Could you check a few things on this model? Use its own coordinates, in mm. A direction names the side the tool comes from. Give positions to 0.01 mm unless a question says otherwise; leave off trailing zeros. Loops run counter-clockwise (first coordinate to the right, second up) from the corner with the lowest first, then second, coordinate; pieces in that order, holes last. Notation, with made-up numbers: (62, 28.25) -> (99, 28.25) arc R19 ccw to (99, 55.25) -> close; hole circle Ø5 at (89.5, 16.25). An arc over 180 degrees is marked (long way). Put each result on its own line as item: value.
```python
from build123d import *

# Parameters (mm, degrees)
SKETCH_1_W          = 130
SKETCH_1_H          = 62
EXTRUDE_1_DEPTH     = 3
SKETCH_2_R          = 2.6
CUT_EXTRUDE_1_DEPTH = 4
SKETCH_3_R          = 1.6
CUT_EXTRUDE_2_DEPTH = 4
CUT_EXTRUDE_3_DEPTH = 4
FILLET_1_R          = 3
FILLET_2_R          = 3


with BuildPart() as part:
    # 草图1 → 凸台-拉伸1 (new body)
    with BuildSketch(Plane.XY):
        Rectangle(SKETCH_1_W, SKETCH_1_H)
    extrude(amount=EXTRUDE_1_DEPTH)

    # 草图2 → 切除-拉伸1 (cut, through all)
    with BuildSketch(Plane.XY.offset(3)):
        with Locations((-45, -26)):
            Circle(SKETCH_2_R)
        with Locations((0, -26)):
            Circle(SKETCH_2_R)
        with Locations((45, -26)):
            Circle(SKETCH_2_R)
    extrude(amount=-CUT_EXTRUDE_1_DEPTH, mode=Mode.SUBTRACT)

    # 草图3 → 切除-拉伸2 (cut, through all)
    with BuildSketch(Plane.XY.offset(3)):
        with Locations((57, 26)):
            Circle(SKETCH_3_R)
        with Locations((57, 6)):
            Circle(SKETCH_3_R)
    cut_extrude_2 = extrude(amount=-CUT_EXTRUDE_2_DEPTH, mode=Mode.SUBTRACT)

    # 镜向1: 切除-拉伸2 across plane
    add(cut_extrude_2.mirror(Plane(origin=(0, 0, 0), x_dir=(0, 0, 1), z_dir=(1, 0, 0))), mode=Mode.SUBTRACT)

    # 草图4 → 切除-拉伸3 (cut, through all)
    with BuildSketch(Plane.XY.offset(3)):
        Polygon((-6.332390824, -19), (-54, 19.840274143), (-54, -19), align=None)
        Polygon((-4, 25), (-47.667609176, 25), (-4, -10.581014884), align=None)
        Polygon((4, 25), (4, -10.581014884), (47.667609176, 25), align=None)
        Polygon((54, 19.840274143), (6.332390824, -19), (54, -19), align=None)
    extrude(amount=-CUT_EXTRUDE_3_DEPTH, mode=Mode.SUBTRACT)

    # 圆角1
    fillet_1_edges = [part.edges().sort_by_distance(p)[0] for p in [
        (-47.667609176, 25, 1.5),
        (-4, 25, 1.5),
        (-4, -10.581014884, 1.5),
        (4, -10.581014884, 1.5),
        (4, 25, 1.5),
        (47.667609176, 25, 1.5),
        (6.332390824, -19, 1.5),
        (54, 19.840274143, 1.5),
        (54, -19, 1.5),
        (-54, 19.840274143, 1.5),
        (-6.332390824, -19, 1.5),
        (-54, -19, 1.5),
    ]]
    fillet(fillet_1_edges, radius=FILLET_1_R)

    # 圆角2
    fillet_2_edges = [part.edges().sort_by_distance(p)[0] for p in [
        (65, -31, 1.5),
        (-65, -31, 1.5),
        (-65, 31, 1.5),
        (65, 31, 1.5),
    ]]
    fillet(fillet_2_edges, radius=FILLET_2_R)


solid = part.part
```
1. If we section it at C-C (x = 57): List the corners of the cut face in (y, z) for me, then the cut area to 3 significant figures.
Recorded:
outline: (-31, 0) -> (4.4, 0) -> (4.4, 3) -> (-31, 3) -> close; (7.6, 0) -> (24.4, 0) -> (24.4, 3) -> (7.6, 3) -> close; (27.6, 0) -> (31, 0) -> (31, 3) -> (27.6, 3) -> close
area: 167 mm^2
2. For faces 1 (the face through (4, 9, 2)), 2 (the face through (65, 0, 1)), which set-ups out of +Z, -Z, +X, -X, +Y, -Y let a thin tool reach every point of the face, with its end or its side?
Recorded:
face 1: +Z, -Z
face 2: +Z, -Z, +X, +Y, -Y
3. Thinking about a two-plate mould opening in X: for faces 3 (the face through (-46.916, -24.243, 1.521)), 4 (the face through (-1, 31, 1)), 5 (the face through (-64.14, -30.1, 1.52)), which applies, pulls with the +X half, pulls with the -X half, needs draft (parallel to the pull), parting line crosses it, or undercut?
Recorded:
face 3: undercut
face 4: needs draft
face 5: pulls with the -X half
4. I'm going to push a flat-ended pin straight in: pin 1 (8.5 mm diameter, centred on x = 45, y = -26, fed in from +Z). Where does the tip first touch, or does it pass through?
Recorded:
pin 1: stops at z = 3
5. I need wall thicknesses on line 1 (Y direction, x = -57, z = 1.5); line 2 (X direction, y = 0, z = 1.05); line 3 (X direction, y = 9.5, z = 1.2). Which ranges of each line are inside material? Lowest first, please.
Recorded:
line 1: y = -31 to 4.4, 7.6 to 24.4, 27.6 to 31
line 2: x = -65 to -54, -29.65 to -16.99, -4 to 4, 16.99 to 29.65, 54 to 65
line 3: x = -65 to -54, -41.31 to -28.64, -4 to 4, 28.64 to 41.31, 54 to 65
6. If we section it at B-B (x = 0): List the corners of the cut face in (y, z) for me, then the cut area to 3 significant figures.
Recorded:
outline: (-31, 0) -> (-28.6, 0) -> (-28.6, 3) -> (-31, 3) -> close; (-23.4, 0) -> (31, 0) -> (31, 3) -> (-23.4, 3) -> close
area: 170 mm^2
7. If we section it at A-A (y = -26): List the corners of the cut face in (x, z) for me.
Recorded:
outline: (-65, 0) -> (-47.6, 0) -> (-47.6, 3) -> (-65, 3) -> close; (-42.4, 0) -> (-2.6, 0) -> (-2.6, 3) -> (-42.4, 3) -> close; (2.6, 0) -> (42.4, 0) -> (42.4, 3) -> (2.6, 3) -> close; (47.6, 0) -> (65, 0) -> (65, 3) -> (47.6, 3) -> close
8. If we section it at D-D (y = 6): List the corners of the cut face in (x, z) for me, then the cut area to 3 significant figures.
Recorded:
outline: (-65, 0) -> (-58.6, 0) -> (-58.6, 3) -> (-65, 3) -> close; (-55.4, 0) -> (-54, 0) -> (-54, 3) -> (-55.4, 3) -> close; (-37.01, 0) -> (-24.35, 0) -> (-24.35, 3) -> (-37.01, 3) -> close; (-4, 0) -> (4, 0) -> (4, 3) -> (-4, 3) -> close; (24.35, 0) -> (37.01, 0) -> (37.01, 3) -> (24.35, 3) -> close; (54, 0) -> (55.4, 0) -> (55.4, 3) -> (54, 3) -> close; (58.6, 0) -> (65, 0) -> (65, 3) -> (58.6, 3) -> close
area: 147 mm^2
